```python
from build123d import *

# Parameters (mm, degrees)
F2_DEPTH = 50.8
F3_DEPTH = 50.8


with BuildPart() as f1:
    # F0 (on Front) → F1 (revolve)
    with BuildSketch(Plane.XZ):
        Polygon((27.0071681589, 56.6442497075), (4.1471673176, 6.4736288041), (4.1471673176, -25.28761141), (23.3657527715, -25.28761141), (23.3657527715, 6.8782302551), (49.8671717942, 56.6442497075), align=None)
    revolve(axis=Axis((4.1471673176, 0, -9.406991303), (0, 0, -1)))

    # F2 (cut): a face of the model
    f2_faces = [f1.faces().sort_by_distance(p)[0] for p in [
        (4.1471673176, 0, -25.28761141),
    ]]
    extrude(f2_faces, amount=-F2_DEPTH, mode=Mode.SUBTRACT)

    # F3 (add): a face of the model
    f3_faces = [f1.faces().sort_by_distance(p)[0] for p in [
        (-14.5278344524, 0, 25.51238859),
    ]]
    extrude(f3_faces, amount=F3_DEPTH)


solid = f1.part
```
CAD build for the part. Positions are in the model's coordinates, mm. Round coordinates to 2 decimals unless told otherwise and drop trailing zeros. Write each loop counter-clockwise with the first axis right and the second up, starting at its lowest first coordinate (ties: lowest second). Pieces come first, ordered by that corner, then holes. Notation, with made-up numbers: (-0.75, 40) - (49.25, 40) arc R30 ccw to (49.25, 62) - close; hole circle Ø5 at (-10.5, -28.75). An arc over 180 degrees is marked (long way). Return JSON: item names as keys, results as strings. Group by question number.
Item 1: Flat gauge pins, fed straight in: pin 1 Ø8 at (x, y) = (-15, 0) entering from +Z; pin 2 Ø10 at (x, z) = (29, 30) entering from -Y; pin 3 Ø10 at (y, z) = (22, 31) entering from +X; pin 4 Ø14 at (x, y) = (4.15, 0) entering from +Z. Where does each tip first touch, or does it go through?
Item 2: Band-saw the part on A-A on y = 0. List the corners of the cut face in (x, z), plus the area to 3 significant figures.
Item 3: Band-saw the part on B-B on z = 32.5. List the corners of the cut face in (x, y), plus the area to 3 significant figures.
Item 4: Mould opens along X. For faces 1 (the face through (2.27, 8.47, 0.47)), 2 (the face through (-11.1, 11.7, -9)), 3 (the face through (-17, 10, 56.644)) say: +X half, -X half, draft (parallel to the pull), parting line (faces both ways), or undercut.
Item 5: Band-saw the part on C-C on z = 12. List the corners of the cut face in (x, y).
Item 6: Probe probe 1 along X at (y, z) = (0, 5); probe 2 along Y at (x, z) = (16, 53.5); probe 3 along Y at (x, z) = (-5, 36.5). List the from-to ranges inside material, lowest first.
Resolved:
{
 "1": {"pin 1": "stops at z = 56.64", "pin 2": "stops at y = -25.75", "pin 3": "stops at x = 32.63", "pin 4": "passes through"},
 "2": {"outline": "(-41.57, 56.64) - (-15.07, 6.88) - (-15.07, -25.29) - (-4.53, -25.29) - (-4.53, 25.51) - (-18.71, 56.64) - close; (12.82, -25.29) - (23.37, -25.29) - (23.37, 6.88) - (49.87, 56.64) - (27.01, 56.64) - (12.82, 25.51) - close", "area": "2,600 mm²"},
 "3": {"outline": "circle Ø65.73 at (4.15, 0); hole circle Ø23.72 at (4.15, 0)", "area": "2,950 mm²"},
 "4": {"face 1": "undercut", "face 2": "parting line", "face 3": "draft"},
 "5": {"outline": "circle Ø43.89 at (4.15, 0); hole circle Ø17.35 at (4.15, 0)"},
 "6": {"probe 1": "x = -15.07 to -4.53, 12.82 to 23.37", "probe 2": "y = -42.42 to -17.85, 17.85 to 42.42", "probe 3": "y = -33.78 to -10.17, 10.17 to 33.78"}
}
